Autodesk Inventor part; units mm, degrees
ref_plane "YZ Plane" through (0, 0, 0) normal (1, 0, 0) x (0, 1, 0)
ref_plane "XZ Plane" through (0, 0, 0) normal (0, 1, 0) x (-1, 0, 0)
ref_plane "XY Plane" through (0, 0, 0) normal (0, 0, 1) x (1, 0, 0)
sketch "Sketch1" plane through (0, 0, 0) normal (0, 1, 0) x (-1, 0, 0)
  line L0 (0, 0) -> (-736.6, 0)
  line L1 (-736.6, 0) -> (-736.6, -812.8)
  line L2 (-736.6, -812.8) -> (0, -812.8)
  line L3 (0, -812.8) -> (0, 0)
  dimension "d0" = 736.6
  dimension "d1" = 812.8
extrude "Extrusion1" add sketch "Sketch1" along normal blind 571.5
sketch "Sketch2" plane through (0, 571.5, 0) normal (0, 1, 0) x (1, 0, 0)
  line L0 (0, 812.8) -> (0, 0)
  line L1 (0, 812.8) -> (88.9, 812.8)
  line L2 (88.9, 812.8) -> (88.9, 574.8444)
  line L3 (88.9, 574.8444) -> (0, 574.8444)
  line L4 (0, 574.8444) -> (0, 812.8)
  dimension "d4" = 88.9
sketch "Sketch7" plane through (0, 571.5, 0) normal (0, 1, 0) x (1, 0, 0)
  line L0 (647.7, 808.0248) -> (90.8173, 808.0248)
  line L1 (90.8173, 808.0248) -> (90.8173, 495.3)
  line L2 (0, 327.5313) -> (279.4, 327.5313)
  line L3 (282.5115, 327.5313) -> (282.5115, 495.3)
  line L4 (279.4, 327.5313) -> (282.5115, 327.5313)
  line L5 (282.5115, 327.5313) -> (0, 327.5313)
  line L6 (647.7, 808.0248) -> (90.8173, 808.0248)
  line L7 (282.5115, 495.3) -> (90.8173, 495.3)
  line L8 (1.5741, 327.5313) -> (1.5741, 4.7643)
  line L9 (1.5741, 4.7643) -> (647.7, 5.5504)
  line L10 (647.7, 808.0248) -> (647.7, 5.5504)
  line L11 (0, 0) -> (736.6, 0)
  point P0 (736.6, 812.8)
extrude "Extrusion7" cut sketch "Sketch7" against normal blind 457.2
sketch "Sketch8" plane through (736.6, 0, 0) normal (1, 0, 0) x (0, 0, -1)
  line L0 (60.9734, 567.6333) -> (749.1017, 567.6333)
  line L1 (749.1017, 567.6333) -> (749.1017, 52.2629)
  line L2 (749.1017, 52.2629) -> (60.9734, 52.2629)
  line L3 (60.9734, 52.2629) -> (60.9734, 567.6333)
  point P0 (0, 0)
extrude "Extrusion8" cut sketch "Sketch8" against normal blind 88.9
sketch "Sketch9" plane through (282.5115, 571.5, -327.5313) normal (1, 0, 0) x (0, 0, -1)
  line L0 (0, 0) -> (0, -457.2)
  line L1 (0, -292.1) -> (167.7687, -292.1)
  line L2 (167.7687, 0) -> (167.7687, -457.2)
  line L3 (421.5704, -457.2) -> (-266.5579, -457.2)
  line L4 (9.1846, -292.1) -> (9.1846, -457.2)
  line L5 (160.1669, -292.1) -> (160.1669, -457.2)
  point P0 (-327.5313, -571.5)
  dimension "d29" = 165.1
extrude "Extrusion9" cut sketch "Sketch9" against normal blind 192.0875 contours L1 L5 L3 L4
sketch "Sketch10" plane through (736.6, 0, -812.8) normal (0, 0, -1) x (-1, 0, 0)
  line L0 (88.9, 571.5) -> (88.9, 114.3)
  line L1 (88.9, 532.7914) -> (711.9203, 532.7914)
  line L2 (711.9203, 532.7914) -> (711.9203, 34.8419)
  line L3 (711.9203, 34.8419) -> (88.9, 34.8419)
  line L4 (88.9, 34.8419) -> (88.9, 532.7914)
  point P0 (736.6, 0)
extrude "Extrusion10" cut sketch "Sketch10" against normal blind 9.525
sketch "Sketch11" plane through (282.5115, 571.5, -495.3) normal (0, 0, -1) x (-1, 0, 0)
  line L0 (0, 0) -> (0, -457.2)
  line L1 (0, -292.1) -> (191.6942, -292.1)
  line L2 (191.6942, 0) -> (191.6942, -457.2)
  line L3 (0, -457.2) -> (191.6942, -457.2)
  line L4 (95.25, -292.1) -> (95.25, -234.95)
  line L5 (0, -292.1) -> (95.25, -234.95)
  line L6 (95.25, -234.95) -> (95.25, -6.35)
  line L7 (95.25, -6.35) -> (0, -6.35)
  point P0 (282.5115, -571.5)
  dimension "d34" = 165.1
  dimension "d35" = 57.15
  dimension "d36" = 95.25
  dimension "d37" = 228.6
extrude "Extrusion11" cut sketch "Sketch11" against normal blind 192.0875 contours L7 L6 L5 L0
sketch "Sketch12" plane through (0, 114.3, 0) normal (0, 1, 0) x (1, 0, 0)
  line L0 (282.5115, 336.7158) -> (460.3115, 336.7158)
  line L1 (460.3115, 336.7158) -> (460.3115, 487.6982)
  line L2 (460.3115, 487.6982) -> (282.5115, 487.6982)
  line L3 (282.5115, 487.6982) -> (282.5115, 336.7158)
  point P0 (0, 0)
  dimension "d40" = 177.8
extrude "Extrusion12" add sketch "Sketch12" along normal blind 139.7
sketch "Sketch13" plane through (460.3115, 114.3, -487.6982) normal (0, 0, -1) x (-1, 0, 0)
  line L0 (0, 0) -> (0, 139.7)
  line L1 (177.8, 165.1) -> (177.8, 0)
  line L2 (0, 139.7) -> (177.8, 0)
  line L3 (0, 122.6899) -> (156.1508, 0)
  line L4 (-187.3885, 0) -> (369.4942, 0)
  point P0 (460.3115, -114.3)
extrude "Extrusion13" cut sketch "Sketch13" against normal blind 188.9125 contours L0 L3 L4
sketch "Sketch14" plane through (460.3115, 254, -487.6982) normal (0, 0, -1) x (-1, 0, 0)
  line L0 (177.8, 0) -> (177.8, -139.7)
  line L1 (0, 0) -> (177.8, -139.7)
  line L2 (458.7374, -139.7) -> (177.8, -139.7)
  line L3 (177.8, -139.7) -> (177.8, 0)
  line L4 (177.8, -139.7) -> (177.8, 0)
  line L5 (0, 0) -> (177.8, 0)
  line L6 (177.8, 0) -> (0, 0)
  point P0 (460.3115, -254)
extrude "Extrusion14" cut sketch "Sketch14" against normal blind 185.7375
properties part number "bot test 1"
Design review of the part built by this model. Coordinates are the model's own, in mm. A direction names the side the tool comes from. Round coordinates to 2 decimals unless told otherwise and drop trailing zeros. Order: outer loops, then holes, each group sorted by start corner. A loop starts at its lowest first (then second) coordinate and runs counter-clockwise, first axis right, second up. Notation, with made-up numbers: M 44,71 L 81,71 A23 cw 81,84 Z; hole C 26,6.25 d6. An arc over 180 degrees is marked long. Put each result on its own line as item: value.
Q1. Machinability: for faces 4 (the face through (234, 565.15, -413)), 5 (the face through (373, 552, -808.025)), 6 (the face through (383.329, 176.504, -413.264)), 7 (the face through (222, 101, -803.275)), 8 (the face through (670, 284, -812.8)), which of the approach directions +Z, -Z, +X, -X, +Y, -Y give a long, thin tool a straight path to every point of the face, cutting with its end or side? Answer none if there is none.
Reported:
face 4: +X
face 5: +Y
face 6: -Z, +X
face 7: -Z
face 8: -Z, +X, -X, +Y, -Y
Q2. Consider section B-B (z = -83.5). State the section outline as (x, y) points.
Reported:
outline: M 0,0 L 736.6,0 L 736.6,52.26 L 647.7,52.26 L 647.7,114.3 L 1.57,114.3 L 1.57,571.5 L 0,571.5 Z; M 647.7,567.63 L 736.6,567.63 L 736.6,571.5 L 647.7,571.5 Z
Q3. To check wall thickness, follow line 1 (Z direction, x = 139, y = 199); line 2 (Z direction, x = 697, y = 103.5); line 3 (Z direction, x = 528, y = 468). State the ranges of each line that lie inside material, in increasing order.
Reported:
line 1: -495.3 to -487.7, -336.72 to -327.53, -4.93 to 0
line 2: -812.8 to -749.1, -60.97 to 0
line 3: -5.4 to 0
Q4. Draft analysis for pull direction Y (two halves, no side actions). For faces 1 (the face through (372.66, 185.13, -413.26)), 2 (the face through (188, 198, -487.698)), 3 (the face through (0, 282, -412)), state which applies: released by +Y, released by -Y, zero draft, split by the parting line, or undercut.
Reported:
face 1: released by +Y
face 2: undercut
face 3: zero draft
Q5. Insertion check: pin 1 Ø3 at (x, y) = (429, 132) entering from -Z; pin 2 Ø4 at (y, z) = (174, -491) entering from +X; pin 3 Ø18.5 at (y, z) = (248, -431) entering from +X. Each pin has a flat end and moves straight along its axis. Give the tip position at first contact, or say it passes through.
Reported:
pin 1: z = -5.29
pin 2: x = 282.51
pin 3: x = 460.31
Q6. Consider section D-D (x = 471). State the section outline as (y, z) points (3 decimals).
Reported:
outline: M 0,-812.8 L 34.842,-812.8 L 34.842,-803.275 L 114.3,-803.275 L 114.3,-5.335 L 571.5,-5.335 L 571.5,0 L 0,0 Z; M 532.791,-812.8 L 571.5,-812.8 L 571.5,-808.025 L 532.791,-808.025 Z
Q7. Consider section A-A (y = 387). State the section outline as (x, z) points (1 decimal), and give its area (3 significant figures).
Reported:
outline: M 0,-812.8 L 24.7,-812.8 L 24.7,-803.3 L 90.8,-803.3 L 90.8,-495.3 L 187.3,-495.3 L 187.3,-327.5 L 1.6,-327.5 L 1.6,-4.8 L 647.7,-5.6 L 647.7,-61 L 736.6,-61 L 736.6,0 L 0,0 Z; M 647.7,-812.8 L 736.6,-812.8 L 736.6,-749.1 L 647.7,-749.1 Z
area: 74,600 mm²
Q8. Consider section C-C (x = 231). State the section outline as (y, z) points (3 decimals), and give its area (3 significant figures).
Reported:
outline: M 0,-812.8 L 34.842,-812.8 L 34.842,-803.275 L 114.3,-803.275 L 114.3,-495.3 L 310.307,-495.3 L 310.307,-327.531 L 114.3,-327.531 L 114.3,-5.043 L 571.5,-5.043 L 571.5,0 L 0,0 Z; M 532.791,-812.8 L 571.5,-812.8 L 571.5,-808.025 L 532.791,-808.025 Z; M 565.15,-495.3 L 571.5,-495.3 L 571.5,-327.531 L 565.15,-327.531 Z; hole M 114.3,-487.698 L 279.4,-487.698 L 279.4,-336.716 L 114.3,-336.716 Z
area: 104,000 mm²
